Study the drawing (mm; zero at the part's minimum x, y, z) and answer. A direction names the side the tool comes from. Round coordinates to 2 decimals unless told otherwise and drop trailing zeros. Loops run counter-clockwise (first coordinate to the right, second up) from the corner with the lowest first, then second, coordinate; pieces in that order, holes last. Notation, with made-up numbers: (0, 68.5) - (20, 68.5) arc R19 cw to (20, 72.5) - close; hole circle Ø6 at (0.5, 4.5). An arc over 180 degrees is marked (long way). Use CSV: the item, a comma, the result in double quotes. Start each with the question number.
1. Determine the mould class of the marked faces 3 and 4 for opening direction Z: +Z half, -Z half, draft (parallel to the pull), parting line (faces both ways), or undercut.
2. Find section A-A (y = 18.5). Give the vertices of the cut face in (x, z).
3. A tool of negligible diameter and unlimited length cuts with its end or side. For the marked faces 1 and 2, from which of +Z, -Z, +X, -X, +Y, -Y can it reach the whole face along a straight path? Write none if from no direction.
4. Find section C-C (x = 1.65). Give the vertices of the cut face in (y, z), and give its area (3 significant figures).
5. Consider line 1 along Y through (x, z) = (1.95, 5); line 2 along Z through (x, y) = (0.6, 21.5). Determine where each line is inside the solid, lowest interval first.
6. Find section B-B (z = 5.75). Give the vertices of the cut face in (x, y).
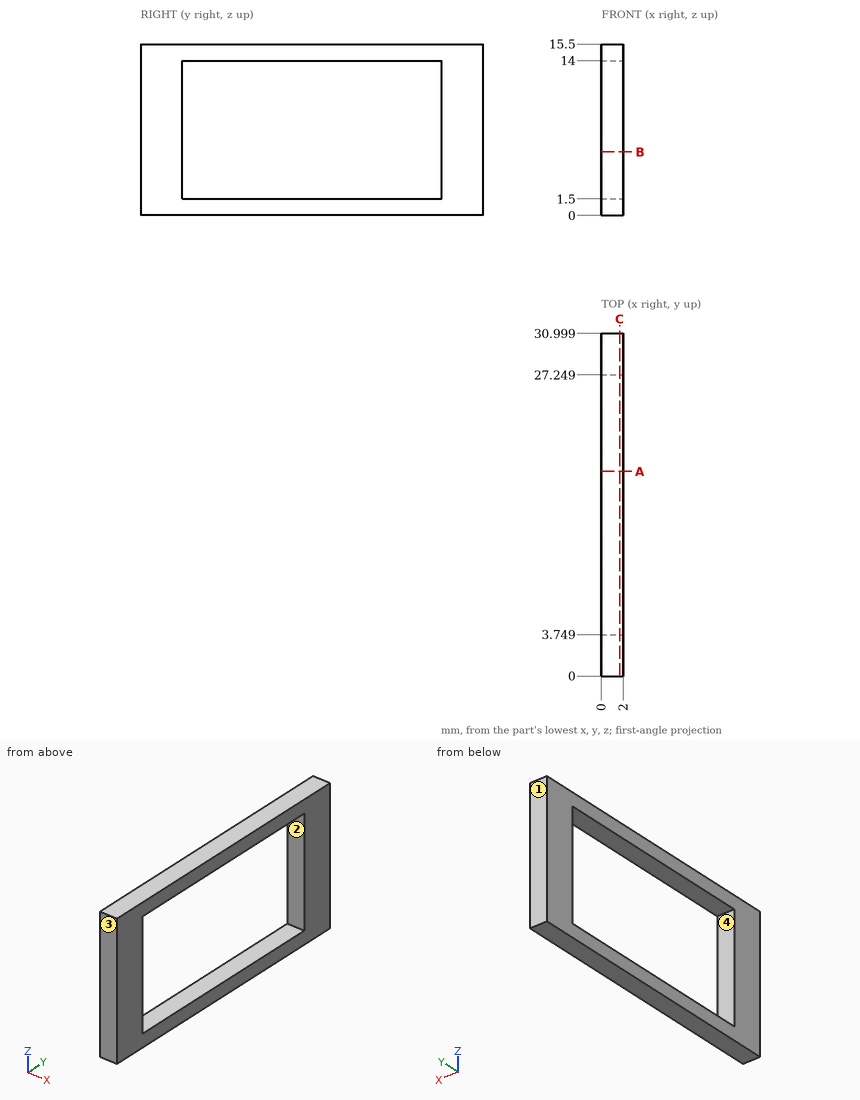
Filled sheet:
1,face 3,"draft"
1,face 4,"undercut"
2,outline,"(0, 0) - (2, 0) - (2, 1.5) - (0, 1.5) - close; (0, 14) - (2, 14) - (2, 15.5) - (0, 15.5) - close"
3,face 1,"+Z, -Z, +X, -X, +Y"
3,face 2,"+X, -X"
4,outline,"(0, 0) - (31, 0) - (31, 15.5) - (0, 15.5) - close; hole (3.75, 1.5) - (27.25, 1.5) - (27.25, 14) - (3.75, 14) - close"
4,area,"187 mm²"
5,line 1,"y = 0 to 3.75, 27.25 to 31"
5,line 2,"z = 0 to 1.5, 14 to 15.5"
6,outline,"(0, 0) - (2, 0) - (2, 3.75) - (0, 3.75) - close; (0, 27.25) - (2, 27.25) - (2, 31) - (0, 31) - close"
